For this review, take the finished solid that the model builds, in its own axes (mm). Round coordinates to 2 decimals unless told otherwise and drop trailing zeros. One line per item, written item: value.
```python
from build123d import *

# Parameters (mm, degrees)
SKETCH_1_R      = 26
SKETCH_1_R_2    = 2
EXTRUDE_1_DEPTH = 3


with BuildPart() as part:
    # Эскиз1 → Вытянуть1 (new body)
    with BuildSketch(Plane.XY):
        with BuildLine():
            ThreePointArc((-5.5, 40.730332677), (-6.779718382, 40.536963609), (-8.052713795, 40.303396886))
            add(Edge.make_bspline(
                [(-18.42711223, 36.737603826), (-9.565846889, 27.871779004), (-8.052713795, 40.303396886)],
                knots=[0, 0, 0, 1, 1, 1], degree=2))
            ThreePointArc((-18.42711223, 36.737603826), (-19.574705107, 36.139188148), (-20.702887125, 35.504935779))
            add(Edge.make_bspline(
                [(-29.357360924, 28.763785557), (-18.097494767, 23.255583732), (-20.702887125, 35.504935779)],
                knots=[0, 0, 0, 1, 1, 1], degree=2))
            ThreePointArc((-29.357360924, 28.763785557), (-30.2484688, 27.825170893), (-31.109581398, 26.858963965))
            add(Edge.make_bspline(
                [(-37.106284036, 17.672964807), (-24.667998276, 16.119285114), (-31.109581398, 26.858963965)],
                knots=[0, 0, 0, 1, 1, 1], degree=2))
            ThreePointArc((-37.106284036, 17.672964807), (-37.644341546, 16.49586462), (-38.145069811, 15.302406645))
            add(Edge.make_bspline(
                [(-40.834165508, 4.667004096), (-28.565341408, 7.236211838), (-38.145069811, 15.302406645)],
                knots=[0, 0, 0, 1, 1, 1], degree=2))
            ThreePointArc((-40.834165508, 4.667004096), (-40.960865773, 3.378975456), (-41.046948028, 2.087596124))
            add(Edge.make_bspline(
                [(-40.137031541, -8.844698925), (-29.367186562, -2.431017271), (-41.046948028, 2.087596124)],
                knots=[0, 0, 0, 1, 1, 1], degree=2))
            ThreePointArc((-40.137031541, -8.844698925), (-39.83864462, -10.104078129), (-39.500752518, -11.353437829))
            add(Edge.make_bspline(
                [(-35.090427416, -21.397941578), (-26.986641373, -11.834807939), (-39.500752518, -11.353437829)],
                knots=[0, 0, 0, 1, 1, 1], degree=2))
            ThreePointArc((-35.090427416, -21.397941578), (-34.399288162, -22.492198068), (-33.674037554, -23.564150627))
            add(Edge.make_bspline(
                [(-26.241230996, -31.632385237), (-21.68167485, -19.95611353), (-33.674037554, -23.564150627)],
                knots=[0, 0, 0, 1, 1, 1], degree=2))
            ThreePointArc((-26.241230996, -31.632385237), (-25.232235072, -32.442939344), (-24.198218116, -33.221322069))
            add(Edge.make_bspline(
                [(-14.548390024, -38.438969129), (-14.027162432, -25.91486457), (-24.198218116, -33.221322069)],
                knots=[0, 0, 0, 1, 1, 1], degree=2))
            ThreePointArc((-14.548390024, -38.438969129), (-13.330877794, -38.877984737), (-12.10014627, -39.278447783))
            add(Edge.make_bspline(
                [(-1.27900525, -41.080094274), (-4.85258931, -29.065337922), (-12.10014627, -39.278447783)],
                knots=[0, 0, 0, 1, 1, 1], degree=2))
            ThreePointArc((-1.27900525, -41.080094274), (0.015086944, -41.099997231), (1.309164177, -41.079144212))
            add(Edge.make_bspline(
                [(12.128979588, -39.269553781), (4.84783716, -29.066130916), (1.309164177, -41.079144212)],
                knots=[0, 0, 0, 1, 1, 1], degree=2))
            ThreePointArc((12.128979588, -39.269553781), (13.359416777, -38.868187292), (14.576606372, -38.428277956))
            add(Edge.make_bspline(
                [(24.222601287, -33.203547806), (14.022925251, -25.917157617), (14.576606372, -38.428277956)],
                knots=[0, 0, 0, 1, 1, 1], degree=2))
            ThreePointArc((24.222601287, -33.203547806), (25.256046509, -32.424406158), (26.264447087, -31.613111508))
            add(Edge.make_bspline(
                [(33.691328284, -23.53942222), (21.678411803, -19.959658145), (26.264447087, -31.613111508)],
                knots=[0, 0, 0, 1, 1, 1], degree=2))
            ThreePointArc((33.691328284, -23.53942222), (34.415791714, -22.466937501), (35.106127425, -21.3721739))
            add(Edge.make_bspline(
                [(39.509077087, -11.324434984), (26.984706061, -11.839220006), (35.106127425, -21.3721739)],
                knots=[0, 0, 0, 1, 1, 1], degree=2))
            ThreePointArc((39.509077087, -11.324434984), (39.846051872, -10.074827555), (40.143514129, -8.815229627))
            add(Edge.make_bspline(
                [(41.045404341, 2.117730498), (29.366788706, -2.435818675), (40.143514129, -8.815229627)],
                knots=[0, 0, 0, 1, 1, 1], degree=2))
            ThreePointArc((41.045404341, 2.117730498), (40.958374033, 3.409046284), (40.830728186, 4.696981559))
            add(Edge.make_bspline(
                [(38.13382515, 15.330407021), (28.566524123, 7.231541404), (40.830728186, 4.696981559)],
                knots=[0, 0, 0, 1, 1, 1], degree=2))
            ThreePointArc((38.13382515, 15.330407021), (37.632220833, 16.523497062), (37.093299291, 17.700201912))
            add(Edge.make_bspline(
                [(31.089854296, 26.881796068), (24.670633395, 16.115251764), (37.093299291, 17.700201912)],
                knots=[0, 0, 0, 1, 1, 1], degree=2))
            ThreePointArc((31.089854296, 26.881796068), (30.228032583, 27.847370544), (29.336235855, 28.785330741))
            add(Edge.make_bspline(
                [(20.676815321, 35.520125397), (18.101296735, 23.252624541), (29.336235855, 28.785330741)],
                knots=[0, 0, 0, 1, 1, 1], degree=2))
            ThreePointArc((20.676815321, 35.520125397), (19.548167965, 36.153549331), (18.400136066, 36.751122333))
            add(Edge.make_bspline(
                [(8.023122571, 40.309297987), (9.570403703, 27.870214648), (18.400136066, 36.751122333)],
                knots=[0, 0, 0, 1, 1, 1], degree=2))
            ThreePointArc((8.023122571, 40.309297987), (6.749956027, 40.541930068), (5.470096027, 40.734359569))
            add(Edge.make_bspline(
                [(-5.5, 40.730332677), (0.00240893, 29.467634546), (5.470096027, 40.734359569)],
                knots=[0, 0, 0, 1, 1, 1], degree=2))
        make_face()
        Circle(SKETCH_1_R, mode=Mode.SUBTRACT)
        with Locations((0, 29.966593386)):
            Circle(SKETCH_1_R_2, mode=Mode.SUBTRACT)
        with Locations((21.189581392, 21.189581392)):
            Circle(SKETCH_1_R_2, mode=Mode.SUBTRACT)
        with Locations((29.966593386, 0)):
            Circle(SKETCH_1_R_2, mode=Mode.SUBTRACT)
        with Locations((21.189581392, -21.189581392)):
            Circle(SKETCH_1_R_2, mode=Mode.SUBTRACT)
        with Locations((0, -29.966593386)):
            Circle(SKETCH_1_R_2, mode=Mode.SUBTRACT)
        with Locations((-21.189581392, -21.189581392)):
            Circle(SKETCH_1_R_2, mode=Mode.SUBTRACT)
        with Locations((-29.966593386, 0)):
            Circle(SKETCH_1_R_2, mode=Mode.SUBTRACT)
        with Locations((-21.189581392, 21.189581392)):
            Circle(SKETCH_1_R_2, mode=Mode.SUBTRACT)
    extrude(amount=EXTRUDE_1_DEPTH)


solid = part.part
```
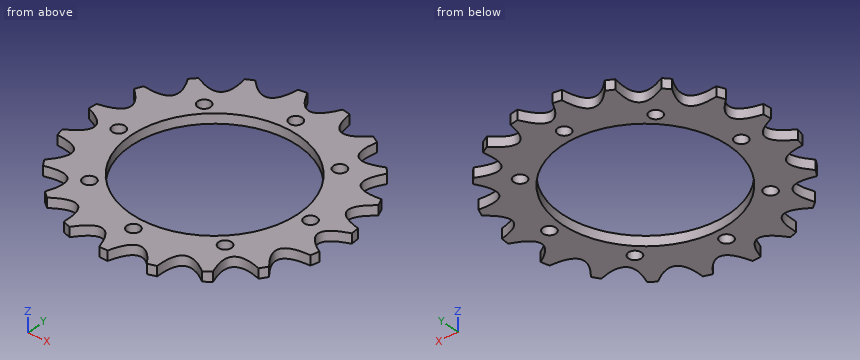
Item 1: Take a section at A-A (x = 0). Count the separate pieces of the cut face and the enclosed holes in it, plus the area to 3 significant figures.
Returned:
separate pieces: 4
enclosed holes: 0
area: 48.6 mm^2
Item 2: For P1, Ø1, axis at y = -19, z = 2, coming from the +X side, flat-tipped, find the tip position at first contact; note if it passes through.
Returned:
P1: x = 33.65
Item 3: Wall thickness on line 1 (Y direction, x = 0, z = 2.05); line 2 (X direction, y = -37, z = 2.15); line 3 (Y direction, x = 35.5, z = 0.8): over which ranges is each line inside the solid? List them lowest first.
Returned:
line 1: -41.1 to -31.97, -27.97 to -26, 26 to 27.97, 31.97 to 35.1
line 2: -14.52 to -10.28, -2.95 to 2.97, 10.31 to 14.55
line 3: -11.84 to -4.84, -1.47 to 6.67, 12.72 to 17.54
